Can you work these out from the model? Positions are in its coordinate system, mm. Face numbers are marked on the shaded views. Round coordinates to 2 decimals unless told otherwise and drop trailing zeros. Loops run counter-clockwise (first coordinate to the right, second up) from the corner with the lowest first, then second, coordinate; pieces in that order, holes last.
```python
from build123d import *

# Parameters (mm, degrees)
ESBO_O1_W                = 75
ESBO_O1_H                = 4
RESSALTO_EXTRUS_O1_DEPTH = 55
ESBO_O4_R                = 1.75
CORTE_EXTRUS_O2_DEPTH    = 5
ESBO_O5_W                = 32
ESBO_O5_H                = 55
ESBO_O5_R                = 1.75
ESBO_O5_W_2              = 25
RESSALTO_EXTRUS_O2_DEPTH = 4
ESBO_O6_R                = 4
CORTE_EXTRUS_O3_DEPTH    = 4
ESBO_O7_W                = 9
ESBO_O7_H                = 55
CORTE_EXTRUS_O4_DEPTH    = 10
FILETE1_R                = 8


with BuildPart() as part:
    # Esboço1 → Ressalto-extrusão1 (new body)
    with BuildSketch(Plane.XY):
        with Locations((37.5, 2)):
            Rectangle(ESBO_O1_W, ESBO_O1_H)
    extrude(amount=RESSALTO_EXTRUS_O1_DEPTH)

    # Esboço4 → Corte-extrusão2 (cut, through all)
    with BuildSketch(Plane.XZ):
        with Locations((50, 7)):
            Circle(ESBO_O4_R)
        with Locations((30, 22.5)):
            Circle(ESBO_O4_R)
        with Locations((30, 42.5)):
            Circle(ESBO_O4_R)
        with Locations((7, 49)):
            Circle(ESBO_O4_R)
        with Locations((7, 6)):
            Circle(ESBO_O4_R)
        with BuildLine():
            Line((51.75, 49.5), (51.75, 46.5))
            ThreePointArc((51.75, 46.5), (50, 44.75), (48.25, 46.5))
            Line((48.25, 46.5), (48.25, 49.5))
            ThreePointArc((48.25, 49.5), (50, 51.25), (51.75, 49.5))
        make_face()
    extrude(amount=-CORTE_EXTRUS_O2_DEPTH, mode=Mode.SUBTRACT)

    # Esboço5 → Ressalto-extrusão2 (add)
    with BuildSketch(Plane(origin=(0, 4, 0), x_dir=(1, 0, 0), z_dir=(0, 1, 0))):
        with Locations((50, -27.5)):
            Rectangle(ESBO_O5_W, ESBO_O5_H)
        with Locations((50, -7)):
            Circle(ESBO_O5_R, mode=Mode.SUBTRACT)
        with BuildLine():
            Line((48.25, -49.5), (48.25, -46.5))
            ThreePointArc((48.25, -46.5), (50, -44.75), (51.75, -46.5))
            Line((51.75, -46.5), (51.75, -49.5))
            ThreePointArc((51.75, -49.5), (50, -51.25), (48.25, -49.5))
        make_face(mode=Mode.SUBTRACT)
        with Locations((12.5, -27.5)):
            Rectangle(ESBO_O5_W_2, ESBO_O5_H)
        with Locations((7, -49)):
            Circle(ESBO_O5_R, mode=Mode.SUBTRACT)
        with Locations((7, -6)):
            Circle(ESBO_O5_R, mode=Mode.SUBTRACT)
    extrude(amount=RESSALTO_EXTRUS_O2_DEPTH)

    # Esboço6 → Corte-extrusão3 (cut)
    with BuildSketch(Plane.XZ):
        with Locations((50, 7)):
            Circle(ESBO_O6_R)
        with Locations((7, 6)):
            Circle(ESBO_O6_R)
        with Locations((7, 49)):
            Circle(ESBO_O6_R)
        with BuildLine():
            Line((46, 46.5), (46, 49.5))
            ThreePointArc((46, 49.5), (50, 53.5), (54, 49.5))
            Line((54, 49.5), (54, 46.5))
            ThreePointArc((54, 46.5), (50, 42.5), (46, 46.5))
        make_face()
    extrude(amount=-CORTE_EXTRUS_O3_DEPTH, mode=Mode.SUBTRACT)

    # Esboço7 → Corte-extrusão4 (cut)
    with BuildSketch(Plane(origin=(0, 4, 0), x_dir=(1, 0, 0), z_dir=(0, 1, 0))):
        with Locations((70.5, -27.5)):
            Rectangle(ESBO_O7_W, ESBO_O7_H)
    extrude(amount=-CORTE_EXTRUS_O4_DEPTH, mode=Mode.SUBTRACT)

    # Filete1
    filete1_edges = [part.edges().sort_by_distance(p)[0] for p in [
        (0, 4, 55),
        (66, 4, 55),
        (66, 4, 0),
        (0, 4, 0),
    ]]
    fillet(filete1_edges, radius=FILETE1_R)


solid = part.part
```
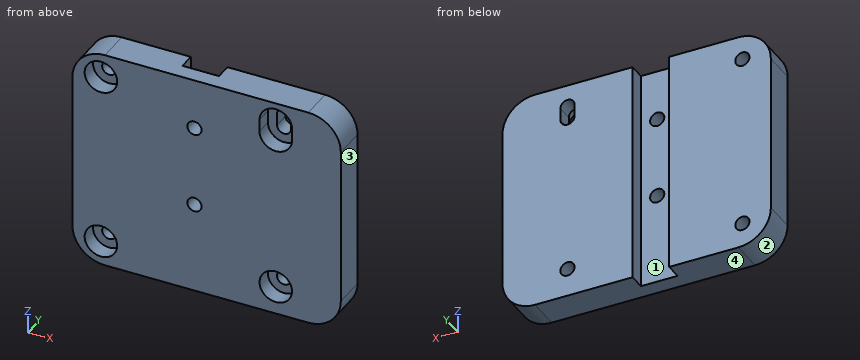
(1) For pin 1 (1.5 mm diameter, centred on y = 1.5, z = 48, fed in from +X); pin 2 (2.5 mm diameter, centred on x = 49.5, z = 8, fed in from -Y); pin 3 (4.5 mm diameter, centred on x = 30, z = 42.5, fed in from +Y), each with a flat end and sliding along its axis, tell me the tip position at first contact or that it passes through.
(2) Suppose I cut it at D-D (y = 2). Write out the boundary of the cut face in (x, z), then the cut area to 3 significant figures.
(3) We'd pull the mould along X, two halves only. Please class the marked faces 1, 2, 3 and 4: released by +X, released by -X, zero draft, split by the parting line, or undercut.
(4) Suppose I cut it at B-B (z = 22.5). Write out the boundary of the cut face in (x, y).
(5) Suppose I cut it at A-A (y = 7). Write out the boundary of the cut face in (x, z).
(6) If I drill on line 1 (Z direction, x = 50, y = 6); line 2 (X direction, y = 6.5, z = 12.5); line 3 (Z direction, x = 30, y = 1.9), over which ranges is the centre line in solid material (lowest first)?
(7) Suppose I cut it at C-C (x = 50). Write out the boundary of the cut face in (y, z).
Check result:
1. pin 1: stops at x = 66
1. pin 2: stops at y = 4
1. pin 3: stops at y = 4
2. outline: (0, 8) arc R8 ccw to (8, 0) - (58, 0) arc R8 ccw to (66, 8) - (66, 47) arc R8 ccw to (58, 55) - (8, 55) arc R8 ccw to (0, 47) - close; hole circle Ø8 at (7, 6); hole circle Ø8 at (7, 49); hole circle Ø3.5 at (30, 22.5); hole circle Ø3.5 at (30, 42.5); hole circle Ø8 at (50, 7); hole (46, 46.5) arc R4 ccw to (54, 46.5) - (54, 49.5) arc R4 ccw to (46, 49.5) - close
2. area: 3,330 mm2
3. face 1: undercut
3. face 2: released by -X
3. face 3: released by +X
3. face 4: zero draft
4. outline: (0, 0) - (28.25, 0) - (28.25, 4) - (25, 4) - (25, 8) - (0, 8) - close; (31.75, 0) - (66, 0) - (66, 8) - (34, 8) - (34, 4) - (31.75, 4) - close
5. outline: (0, 8) arc R8 ccw to (8, 0) - (25, 0) - (25, 55) - (8, 55) arc R8 ccw to (0, 47) - close; (34, 0) - (58, 0) arc R8 ccw to (66, 8) - (66, 47) arc R8 ccw to (58, 55) - (34, 55) - close; hole circle Ø3.5 at (7, 6); hole circle Ø3.5 at (7, 49); hole circle Ø3.5 at (50, 7); hole (48.25, 46.5) arc R1.75 ccw to (51.75, 46.5) - (51.75, 49.5) arc R1.75 ccw to (48.25, 49.5) - close
6. line 1: z = 0 to 5.25, 8.75 to 44.75, 51.25 to 55
6. line 2: x = 0 to 25, 34 to 66
6. line 3: z = 0 to 20.75, 24.25 to 40.75, 44.25 to 55
7. outline: (0, 0) - (8, 0) - (8, 5.25) - (4, 5.25) - (4, 3) - (0, 3) - close; (0, 11) - (4, 11) - (4, 8.75) - (8, 8.75) - (8, 44.75) - (4, 44.75) - (4, 42.5) - (0, 42.5) - close; (0, 53.5) - (4, 53.5) - (4, 51.25) - (8, 51.25) - (8, 55) - (0, 55) - close
